```python
from build123d import *

# Parameters (mm, degrees)
F1_DEPTH = 2


# Not quite as in the source:
# - ends of sketch curves that miss each other by under 0.0002 mm in the source are joined
# - the dataset's text gives a spline's control points without its knots; the knots are read off the source's solid


with BuildPart() as f1:
    # F0 (on Top) → F1 (new body)
    with BuildSketch(Plane.XY):
        with BuildLine():
            add(Edge.make_bspline(
                [(-4.5539323159, 3.4404925622), (-4.553932314, 4.109133441), (-4.4417509068, 4.6815041688), (-4.121937897, 5.4234547922), (-3.9898413305, 5.6517314099), (-3.6715155244, 6.0768112467), (-3.4851703783, 6.273694276), (-3.2685167558, 6.4563475141)],
                knots=[0, 0, 0, 0, 0.5, 0.5, 0.75, 0.75, 1, 1, 1, 1], degree=3))
            add(Edge.make_bspline(
                [(-4.1653522884, 1.6684308192), (-4.4188295054, 2.1571348906), (-4.5539323132, 2.7395984093), (-4.5539323159, 3.4404925622)],
                knots=[0, 0, 0, 0, 1, 1, 1, 1], degree=3))
            add(Edge.make_bspline(
                [(-3.0880831784, 0.3100080442), (-3.5410735232, 0.7013744056), (-3.8969951229, 1.1510382057), (-4.1653522884, 1.6684308192)],
                knots=[0, 0, 0, 0, 1, 1, 1, 1], degree=3))
            add(Edge.make_bspline(
                [(-0.94726724, -0.9733503247), (-0.9476283907, -0.9731801173), (-0.9479895414, -0.9730099099), (-0.948350692, -0.9728397025), (-1.4381555261, -0.7419986681), (-1.8627330629, -0.5176434714), (-2.5774559291, -0.0871012519), (-2.8674308006, 0.1193728081), (-3.0880831784, 0.3100080442)],
                knots=[-0.0003686679, -0.0003686679, -0.0003686679, -0.0003686679, 0, 0, 0, 0.5, 0.5, 1, 1, 1, 1], degree=3))
            add(Edge.make_bspline(
                [(1.2638188496, -2.1313058458), (1.0591492674, -1.9955628295), (0.7810896534, -1.8386696922), (0.0493295513, -1.4564253852), (-0.4034193402, -1.2324993239), (-0.9461859739, -0.9738655589), (-0.9465463959, -0.9736938141), (-0.946906818, -0.9735220694), (-0.94726724, -0.9733503247)],
                knots=[0, 0, 0, 0, 0.5, 0.5, 1, 1, 1, 1.000332023, 1.000332023, 1.000332023, 1.000332023], degree=3))
            add(Edge.make_bspline(
                [(2.2073726786, -3.0012041242), (1.9740381312, -2.6745358034), (1.654810322, -2.3906232081), (1.2638188496, -2.1313058458)],
                knots=[0, 0, 0, 0, 1, 1, 1, 1], degree=3))
            add(Edge.make_bspline(
                [(2.5831118874, -4.1916276187), (2.5831119009, -3.9779409831), (2.5527095247, -3.7664931745), (2.4264212856, -3.3640546657), (2.3305505576, -3.173653134), (2.2073726786, -3.0012041242)],
                knots=[0, 0, 0, 0, 0.5, 0.5, 1, 1, 1, 1], degree=3))
            add(Edge.make_bspline(
                [(1.7310564521, -5.9594051259), (1.8694470021, -5.8607866548), (1.9951638757, -5.7464648732), (2.2124688094, -5.4892251058), (2.3038523063, -5.3464167266), (2.519150799, -4.8886706939), (2.5831119027, -4.5468724456), (2.5831118874, -4.1916276187)],
                knots=[0, 0, 0, 0, 0.25, 0.25, 0.5, 0.5, 1, 1, 1, 1], degree=3))
            add(Edge.make_bspline(
                [(-0.3604753147, -6.502818499), (0.0582122658, -6.5028185014), (0.4414416098, -6.4634017893), (1.1407820285, -6.2894614297), (1.4577253675, -6.1541835635), (1.7310564521, -5.9594051259)],
                knots=[0, 0, 0, 0, 0.5, 0.5, 1, 1, 1, 1], degree=3))
            add(Edge.make_bspline(
                [(-2.6224302874, -6.1809013634), (-1.8135993387, -6.3928882585), (-1.0605109021, -6.5028184969), (-0.3604753147, -6.502818499)],
                knots=[0, 0, 0, 0, 1, 1, 1, 1], degree=3))
            add(Edge.make_bspline(
                [(-4.7454580591, -5.4407007971), (-3.9473161615, -5.7716151358), (-3.2419123285, -6.018541014), (-2.6224302874, -6.1809013634)],
                knots=[0.2417760748, 0.2417760748, 0.2417760748, 0.2417760748, 1, 1, 1, 1], degree=3))
            Line((-4.7454580591, -5.4407007971), (-4.7454580591, -7.4795386684))
            add(Edge.make_bspline(
                [(-0.6315023097, -8.2730601286), (-2.1864345754, -8.2730601282), (-3.5521940185, -8.0048830709), (-4.7454580591, -7.4795386684)],
                knots=[0, 0, 0, 0, 0.9183123613, 0.9183123613, 0.9183123613, 0.9183123613], degree=3))
            add(Edge.make_bspline(
                [(3.4928160756, -7.1080140655), (3.0203241877, -7.4861136355), (2.4493404192, -7.7758563937), (1.0800859896, -8.1699938198), (0.2819186052, -8.2730601281), (-0.6315023097, -8.2730601286)],
                knots=[0, 0, 0, 0, 0.5, 0.5, 1, 1, 1, 1], degree=3))
            add(Edge.make_bspline(
                [(4.8917938139, -4.0217840352), (4.8917938118, -4.7009415685), (4.7711067522, -5.2821953174), (4.4246282935, -6.0408703732), (4.2811707681, -6.2753258521), (3.9340237801, -6.7139024983), (3.7301988047, -6.918054596), (3.4928160756, -7.1080140655)],
                knots=[0, 0, 0, 0, 0.5, 0.5, 0.75, 0.75, 1, 1, 1, 1], degree=3))
            add(Edge.make_bspline(
                [(4.1507940458, -1.638882878), (4.396515413, -1.9570273867), (4.5792206673, -2.30751695), (4.827118095, -3.0950479417), (4.8917938123, -3.5328168935), (4.8917938139, -4.0217840352)],
                knots=[0, 0, 0, 0, 0.5, 0.5, 1, 1, 1, 1], degree=3))
            add(Edge.make_bspline(
                [(1.1782471579, 0.4183491959), (1.9294970419, 0.0585462091), (2.5547792836, -0.2982557111), (3.5466215561, -0.992037242), (3.9119064629, -1.3295863067), (4.1507940458, -1.638882878)],
                knots=[0, 0, 0, 0, 0.5, 0.5, 1, 1, 1, 1], degree=3))
            add(Edge.make_bspline(
                [(-1.1143311666, 1.6184455474), (-1.0162509018, 1.5510390918), (-0.9004048855, 1.4804604262), (-0.6206808382, 1.3208013117), (-0.45698794, 1.2321520315), (0.1108160421, 0.9359869549), (0.5914968065, 0.6983949543), (1.1782471579, 0.4183491959)],
                knots=[0, 0, 0, 0, 0.25, 0.25, 0.5, 0.5, 0.9998046197, 0.9998046197, 0.9998046197, 0.9998046197], degree=3))
            add(Edge.make_bspline(
                [(-1.9560474883, 2.451198266), (-1.8566181148, 2.2916099906), (-1.7343676506, 2.1446246375), (-1.4523338231, 1.8693058849), (-1.2924097348, 1.7408315854), (-1.1143311666, 1.6184455474)],
                knots=[0, 0, 0, 0, 0.5, 0.5, 1, 1, 1, 1], degree=3))
            add(Edge.make_bspline(
                [(-2.2560914692, 3.5561307467), (-2.2560914812, 3.358554546), (-2.232979569, 3.1644905564), (-2.1338539681, 2.7921448588), (-2.0575762287, 2.6141561535), (-1.9560474883, 2.451198266)],
                knots=[0, 0, 0, 0, 0.5, 0.5, 1, 1, 1, 1], degree=3))
            add(Edge.make_bspline(
                [(-1.5318803699, 5.1870673998), (-1.6485374043, 5.0854884976), (-1.7539534558, 4.9731201094), (-1.9368474168, 4.7284320339), (-2.0142254381, 4.5961241937), (-2.1985253422, 4.1773747627), (-2.2560914855, 3.8703955411), (-2.2560914692, 3.5561307467)],
                knots=[0, 0, 0, 0, 0.25, 0.25, 0.5, 0.5, 1, 1, 1, 1], degree=3))
            add(Edge.make_bspline(
                [(0.3622633388, 5.7878203751), (-0.012208003, 5.7878203799), (-0.3599577221, 5.7447623809), (-0.9981166165, 5.5511975822), (-1.2885907071, 5.398911453), (-1.5318803699, 5.1870673998)],
                knots=[0, 0, 0, 0, 0.5, 0.5, 1, 1, 1, 1], degree=3))
            add(Edge.make_bspline(
                [(2.1965066912, 5.556154833), (1.5795493196, 5.7097488235), (0.967120358, 5.7878203748), (0.3622633388, 5.7878203751)],
                knots=[0, 0, 0, 0, 1, 1, 1, 1], degree=3))
            add(Edge.make_bspline(
                [(3.9397827582, 4.9814492737), (3.2685520169, 5.2415958191), (2.6904101659, 5.4331955967), (2.1965066912, 5.556154833)],
                knots=[0.1998130955, 0.1998130955, 0.1998130955, 0.1998130955, 1, 1, 1, 1], degree=3))
            Line((3.9397827582, 4.9814492737), (4.6406248453, 6.6751509842))
            add(Edge.make_bspline(
                [(2.7885063884, 7.2906242127), (3.380503744, 7.1369061979), (3.9980767952, 6.9320131673), (4.6406248453, 6.6751509842)],
                knots=[0, 0, 0, 0, 0.7923628244, 0.7923628244, 0.7923628244, 0.7923628244], degree=3))
            add(Edge.make_bspline(
                [(0.4742878301, 7.5761304711), (1.2877472267, 7.5761304708), (2.0577984223, 7.4803598207), (2.7885063884, 7.2906242127)],
                knots=[0, 0, 0, 0, 1, 1, 1, 1], degree=3))
            add(Edge.make_bspline(
                [(-3.2685167558, 6.4563475141), (-2.836280375, 6.8207511786), (-2.3183058122, 7.0983331165), (-1.0776039847, 7.4767690155), (-0.3546345611, 7.5761304704), (0.4742878301, 7.5761304711)],
                knots=[0, 0, 0, 0, 0.5, 0.5, 1, 1, 1, 1], degree=3))
        make_face()
    extrude(amount=F1_DEPTH)


solid = f1.part
```
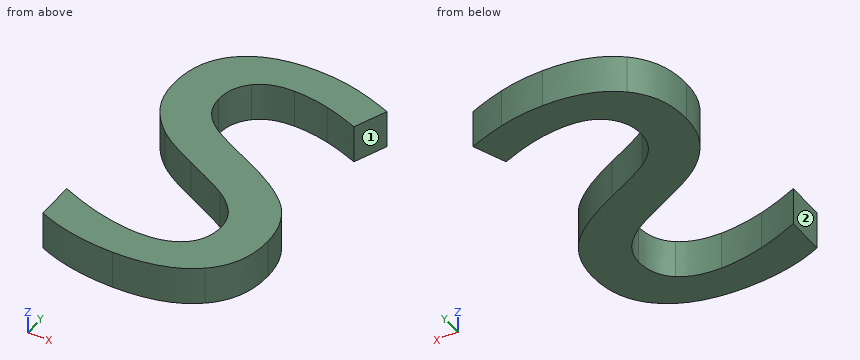
Check sheet for the modelled part. Datum: model origin and axes. Units: mm. Face numbers are marked on the shaded views. Give positions to 0.01 mm unless a question says otherwise; leave off trailing zeros.
Item 1: Scan lines: L1, parallel to Y at x = -1, z = 0.6; L2, parallel to Y at x = 0, z = 1.5; L3, parallel to Y at x = -3.5, z = 0.2. Record each from-to range of solid material in increasing order.
Item 2: Cross-section at A-A (x = 1.5). Count the separate pieces of the cut face and the enclosed holes in it, and give its area (3 significant figures).
Item 3: Draft check along Y on the marked faces 1 and 2. Enter one of: released by +Y, released by -Y, zero draft, split by the parting line, or undercut.
Item 4: Gauge pin test, flat end, axial feed: pin 1 (1 mm diameter, centred on y = 0, z = 1, fed in from +X). Record the tip position at first contact, or that the pin passes through.
Report:
1. L1: y = -8.27 to -6.47, -0.95 to 1.54, 5.53 to 7.45
1. L2: y = -8.26 to -6.49, -1.44 to 1, 5.77 to 7.56
1. L3: y = -7.92 to -5.91, 0.71 to 6.24
2. separate pieces: 3
2. enclosed holes: 0
2. area: 12.6 mm2
3. face 1: undercut
3. face 2: zero draft
4. pin 1: stops at x = 2.84
